from build123d import *

# Parameters (mm, degrees)
SKETCH1_W           = 70
SKETCH1_H           = 70
BOSS_EXTRUDE1_DEPTH = 39
CHAMFER1_SIZE       = 5
SHELL1_T            = -2
SKETCH3_W           = 2.5
SKETCH3_H           = 66
BOSS_EXTRUDE2_DEPTH = 5


with BuildPart() as part:
    # Sketch1 → Boss-Extrude1 (new body)
    with BuildSketch(Plane.XY):
        with Locations((86.822194683, -0.073375262)):
            Rectangle(SKETCH1_W, SKETCH1_H)
    extrude(amount=-BOSS_EXTRUDE1_DEPTH)

    # Chamfer1
    chamfer1_edges = [part.edges().sort_by_distance(p)[0] for p in [
        (51.822194683, 34.926624738, -19.5),
        (121.822194683, 34.926624738, -19.5),
        (121.822194683, -35.073375262, -19.5),
        (51.822194683, -35.073375262, -19.5),
    ]]
    chamfer(chamfer1_edges, length=CHAMFER1_SIZE)

    # Shell1
    shell1_openings = [part.faces().sort_by_distance(p)[0] for p in [
        (86.822194683, -0.073375262, 0),
    ]]
    offset(amount=SHELL1_T, openings=shell1_openings, kind=Kind.INTERSECTION)

    # Sketch3 → Boss-Extrude2 (add)
    with BuildSketch(Plane.XY.offset(-37)):
        with Locations((68.572194683, -0.073375262)):
            Rectangle(SKETCH3_W, SKETCH3_H)
        with Locations((105.072194683, -0.073375262)):
            Rectangle(SKETCH3_W, SKETCH3_H)
    extrude(amount=BOSS_EXTRUDE2_DEPTH)


solid = part.part
Read the model definition and answer for the solid it produces. Units are mm, in the model's axes. A direction names the side the tool comes from. Give positions to 0.01 mm unless a question says otherwise; leave off trailing zeros. Loops run counter-clockwise (first coordinate to the right, second up) from the corner with the lowest first, then second, coordinate; pieces in that order, holes last. Notation, with made-up numbers: (-2.5, 25.5) -> (20.5, 25.5) arc R24 ccw to (20.5, 56.5) -> close; hole circle Ø8 at (11.5, 26). An arc over 180 degrees is marked (long way). Use a Markdown table: item, result.
Q1. Determine the mould class of faces 1 (the face through (87, -34, 0)), 2 (the face through (55.763, 31.039, -18.241)), 3 (the face through (54.36, -32.61, -19.23)) for opening direction Y: pulls with the +Y half, pulls with the -Y half, needs draft (parallel to the pull), parting line crosses it, or undercut.
Solved:
| item | result |
|---|---|
| face 1 | needs draft |
| face 2 | undercut |
| face 3 | pulls with the -Y half |
Q2. Section A-A, the plane z = -33 is taken. Determine the outline of the cut face in (x, y).
Solved:
| item | result |
|---|---|
| outline | (51.82, -30.07) -> (56.82, -35.07) -> (116.82, -35.07) -> (121.82, -30.07) -> (121.82, 29.93) -> (116.82, 34.93) -> (56.82, 34.93) -> (51.82, 29.93) -> close; hole (53.82, -29.24) -> (57.65, -33.07) -> (67.32, -33.07) -> (67.32, 32.93) -> (57.65, 32.93) -> (53.82, 29.1) -> close; hole (69.82, -33.07) -> (103.82, -33.07) -> (103.82, 32.93) -> (69.82, 32.93) -> close; hole (106.32, -33.07) -> (115.99, -33.07) -> (119.82, -29.24) -> (119.82, 29.1) -> (115.99, 32.93) -> (106.32, 32.93) -> close |
Q3. Section B-B, the plane z = -27 is taken. Determine the outline of the cut face in (x, y), then the cut area to 3 significant figures.
Solved:
| item | result |
|---|---|
| outline | (51.82, -30.07) -> (56.82, -35.07) -> (116.82, -35.07) -> (121.82, -30.07) -> (121.82, 29.93) -> (116.82, 34.93) -> (56.82, 34.93) -> (51.82, 29.93) -> close; hole (53.82, -29.24) -> (57.65, -33.07) -> (115.99, -33.07) -> (119.82, -29.24) -> (119.82, 29.1) -> (115.99, 32.93) -> (57.65, 32.93) -> (53.82, 29.1) -> close |
| area | 523 mm^2 |
Q4. Find the intervals of material crossed by line 1 along X through (y, z) = (-6, -36); line 2 along Y through (x, z) = (64, -31.5); line 3 along X through (y, z) = (-11, -12), in increasing order.
Solved:
| item | result |
|---|---|
| line 1 | x = 51.82 to 53.82, 67.32 to 69.82, 103.82 to 106.32, 119.82 to 121.82 |
| line 2 | y = -35.07 to -33.07, 32.93 to 34.93 |
| line 3 | x = 51.82 to 53.82, 119.82 to 121.82 |
Q5. Section C-C, the plane x = 75 is taken. Determine the outline of the cut face in (y, z).
Solved:
| item | result |
|---|---|
| outline | (-35.07, -39) -> (34.93, -39) -> (34.93, 0) -> (32.93, 0) -> (32.93, -37) -> (-33.07, -37) -> (-33.07, 0) -> (-35.07, 0) -> close |
Q6. A tool of negligible diameter and unlimited length cuts with its end or side. For faces 4 (the face through (119.29, 32.46, -19.23)), 5 (the face through (106.322, -1, -35)), from which of +Z, -Z, +X, -X, +Y, -Y can it reach the whole face along a straight path? Write none if from no direction.
Solved:
| item | result |
|---|---|
| face 4 | +Z, -Z, +X, +Y |
| face 5 | +Z |
Q7. Each of these flat-tipped pins is pushed along its axis until it touches: pin 1 (2 mm diameter, centred on x = 105.5, y = -1.5, fed in from +Z); pin 2 (7 mm diameter, centred on x = 115.5, y = -2.5, fed in from +Z). Where does it stop, or does it pass through?
Solved:
| item | result |
|---|---|
| pin 1 | stops at z = -32 |
| pin 2 | stops at z = -37 |
Q8. Section D-D, the plane y = 0.5 is taken. Determine the outline of the cut face in (x, z), then the cut area to 3 significant figures.
Solved:
| item | result |
|---|---|
| outline | (51.82, -39) -> (121.82, -39) -> (121.82, 0) -> (119.82, 0) -> (119.82, -37) -> (106.32, -37) -> (106.32, -32) -> (103.82, -32) -> (103.82, -37) -> (69.82, -37) -> (69.82, -32) -> (67.32, -32) -> (67.32, -37) -> (53.82, -37) -> (53.82, 0) -> (51.82, 0) -> close |
| area | 313 mm^2 |
